```python
from build123d import *

# Parameters (mm, degrees)
SKETCH1_W           = 41
SKETCH1_H           = 41
BOSS_EXTRUDE1_DEPTH = 12.5
SKETCH2_W           = 10
SKETCH2_H           = 1.5
CUT_EXTRUDE1_DEPTH  = 5
SKETCH3_W           = 7
SKETCH3_H           = 4
CUT_EXTRUDE2_DEPTH  = 5
SKETCH4_W           = 15
SKETCH4_H           = 5
CUT_EXTRUDE3_DEPTH  = 5
SKETCH5_W           = 11
SKETCH5_H           = 4
BOSS_EXTRUDE2_DEPTH = 5


with BuildPart() as part:
    # Sketch1 → Boss-Extrude1 (new body)
    with BuildSketch(Plane(origin=(0, 0, 0), x_dir=(1, 0, 0), z_dir=(0, 1, 0))):
        with Locations((20.5, 20.5)):
            Rectangle(SKETCH1_W, SKETCH1_H)
    extrude(amount=BOSS_EXTRUDE1_DEPTH)

    # Sketch2 → Cut-Extrude1 (cut)
    with BuildSketch(Plane.XY):
        with Locations((10.5, 11.75)):
            Rectangle(SKETCH2_W, SKETCH2_H)
    extrude(amount=-CUT_EXTRUDE1_DEPTH, mode=Mode.SUBTRACT)

    # Sketch3 → Cut-Extrude2 (cut)
    with BuildSketch(Plane.XY):
        with Locations((6, 4)):
            Rectangle(SKETCH3_W, SKETCH3_H)
    extrude(amount=-CUT_EXTRUDE2_DEPTH, mode=Mode.SUBTRACT)

    # Sketch4 → Cut-Extrude3 (cut)
    with BuildSketch(Plane.XY):
        with Locations((28, 5.5)):
            Rectangle(SKETCH4_W, SKETCH4_H)
    extrude(amount=-CUT_EXTRUDE3_DEPTH, mode=Mode.SUBTRACT)

    # Sketch5 → Boss-Extrude2 (add)
    with BuildSketch(Plane(origin=(0, 0, -41), x_dir=(-1, 0, 0), z_dir=(0, 0, -1))):
        with Locations((-33, 5.5)):
            Rectangle(SKETCH5_W, SKETCH5_H)
    extrude(amount=BOSS_EXTRUDE2_DEPTH)


solid = part.part
```
Check sheet for the modelled part. Datum: model origin and axes. Units: mm. A direction names the side the tool comes from. Coordinates: 2 decimals unless noted, no trailing zeros. Loops run counter-clockwise (first coordinate to the right, second up) from the corner with the lowest first, then second, coordinate; pieces in that order, holes last. Notation, with made-up numbers: M 36,7 L 85,7 A27 ccw 85,33 Z; hole C 9.5,75.25 d5. An arc over 180 degrees is marked long. Answer as a JSON object with one key per item and string values.
1. Sectioned sample at D-D on x = 31.5. Record the cut outline in (y, z).
Outcome:
{"outline": "M 0,-41 L 3.5,-41 L 3.5,-46 L 7.5,-46 L 7.5,-41 L 12.5,-41 L 12.5,0 L 8,0 L 8,-5 L 3,-5 L 3,0 L 0,0 Z"}
2. Scan lines: L1, parallel to Y at x = 35, z = -2; L2, parallel to X at y = 7, z = -44; L3, parallel to Z at x = 21, y = 3.25. Record each from-to range of solid material in increasing order. Write a range as from..to.
Outcome:
{"L1": "0..3, 8..12.5", "L2": "27.5..38.5", "L3": "-41..-5"}
3. Sectioned sample at A-A on z = -4. Record the cut outline in (x, y), and give its area (4 significant figures).
Outcome:
{"outline": "M 0,0 L 41,0 L 41,12.5 L 15.5,12.5 L 15.5,11 L 5.5,11 L 5.5,12.5 L 0,12.5 Z; hole M 2.5,2 L 9.5,2 L 9.5,6 L 2.5,6 Z; hole M 20.5,3 L 35.5,3 L 35.5,8 L 20.5,8 Z", "area": "394.5 mm²"}
4. Release check for a two-part mould opening along Y. For faces 1 (the flat face through (9.5, 4, -2)), 2 (the flat face through (27.5, 5, -43)), 3 (the flat face through (33, 7.5, -43)) record: pulls with the +Y half, pulls with the -Y half, needs draft (parallel to the pull), parting line crosses it, or undercut.
Outcome:
{"face 1": "undercut", "face 2": "needs draft", "face 3": "pulls with the +Y half"}
5. Sectioned sample at B-B on x = 36.5. Record the cut outline in (y, z).
Outcome:
{"outline": "M 0,-41 L 3.5,-41 L 3.5,-46 L 7.5,-46 L 7.5,-41 L 12.5,-41 L 12.5,0 L 0,0 Z"}
6. Depth check by flat-ended pin: P1, Ø1.5, axis at y = 9.5, z = -27, coming from the -X side; P2, Ø2.5, axis at x = 30, y = 4.5, coming from the +Z side; P3, Ø1.5, axis at x = 10, z = -3, coming from the +Y side; P4, Ø2, axis at x = 5.5, y = 2.5, coming from the -Z side. Enter the tip coordinate at first touch or a pass-through.
Outcome:
{"P1": "x = 0", "P2": "z = -5", "P3": "y = 11", "P4": "z = -41"}
7. Sectioned sample at C-C on y = 10.25. Record the cut outline in (x, z), and give its area (3 significant figures).
Outcome:
{"outline": "M 0,-41 L 41,-41 L 41,0 L 0,0 Z", "area": "1,680 mm²"}
8. Access from +Z, -Z, +X, -X, +Y, -Y to the whole of each face (thin tool, end or side, straight path). Record for faces 4 (the flat face through (2.5, 4, -2)), 5 (the flat face through (38.5, 5, -43)), 6 (the flat face through (33, 3.5, -43)), 7 (the flat face through (10, 11, -2)).
Outcome:
{"face 4": "+Z", "face 5": "-Z, +X, +Y, -Y", "face 6": "-Z, +X, -X, -Y", "face 7": "+Z, +Y"}
